Geometry check sheet. Reference: the model listing, model coordinates, mm. A direction names the side the tool comes from. Coordinates: 2 decimals unless noted, no trailing zeros. Loops run counter-clockwise (first coordinate to the right, second up) from the corner with the lowest first, then second, coordinate; pieces in that order, holes last. Notation, with made-up numbers: M 49.25,-24.5 L 105.25,-24.5 A22 cw 105.25,-17.5 Z; hole C 4,5 d9. An arc over 180 degrees is marked long. Use CSV: the item, a comma, the result in double quotes.
```python
from build123d import *

# Parameters (mm, degrees)
F0_R     = 25.4
F0_W     = 3.81
F0_H     = 19.05
F1_DEPTH = 3.429


# Not quite as in the source:
# - ends of sketch curves that miss each other by under 0.0002 mm in the source are joined


with BuildPart() as f1:
    # F0 (on Front) → F1 (new body)
    with BuildSketch(Plane.XZ):
        with BuildLine():
            ThreePointArc((-642.1692497265, -473.1768646252), (-619.4825639758, -474.3339275445), (-599.5683960075, -485.2632650852))
            ThreePointArc((-599.5683960075, -485.2632650852), (-473.9081608396, -561.5426017902), (-329.3321582, -588.1285164))
            Line((-329.3321582, -588.1285164), (312.391679, -588.1285164))
            ThreePointArc((312.391679, -588.1285164), (370.7126340924, -576.5277571547), (420.1547524528, -543.4915898528))
            Line((420.1547524528, -543.4915898528), (432.6678418, -530.9785164))
            Line((432.6678418, -530.9785164), (432.6678418, -518.2785164))
            Line((432.6678418, -518.2785164), (115.1678418, -518.2785164))
            Line((115.1678418, -518.2785164), (115.1678418, -486.5285164))
            Line((115.1678418, -486.5285164), (-329.3321582, -486.5285164))
            ThreePointArc((-329.3321582, -486.5285164), (-500.4183293998, -433.9834708096), (-612.5167665735, -294.4650126217))
            Line((-612.5167665735, -294.4650126217), (-633.7122454, -241.2238))
            ThreePointArc((-633.7122454, -241.2238), (-715.4828245955, -108.0397407431), (-837.3321571082, -10.1767620246))
            Line((-837.3321571082, -10.1767620246), (-888.1321582, -98.1649548))
            ThreePointArc((-888.1321582, -98.1649548), (-792.2711581527, -174.5413586603), (-728.0333576386, -278.9261845185))
            Line((-728.0333576386, -278.9261845185), (-706.971662, -331.8929862))
            ThreePointArc((-706.971662, -331.8929862), (-701.288086285, -345.465340488), (-695.1169115223, -358.8230511462))
            ThreePointArc((-695.1169115223, -358.8230511462), (-695.6103607346, -404.0881567784), (-732.0186808394, -430.9880994311))
            Line((-732.0186808394, -430.9880994311), (-778.7941498, -439.2359008))
            ThreePointArc((-778.7941498, -439.2359008), (-797.5979576606, -451.5111596623), (-801.724697479, -473.5845717908))
            Line((-801.724697479, -473.5845717908), (-659.172037, -448.448684))
            Line((-659.172037, -448.448684), (-658.5104432, -452.2007974))
            Line((-658.5104432, -452.2007974), (-800.6426456, -477.2625456))
            ThreePointArc((-800.6426456, -477.2625456), (-788.0677244467, -492.1533513081), (-768.8701676538, -495.5176466233))
            Line((-768.8701676538, -495.5176466233), (-642.1692497265, -473.1768646252))
        make_face()
        Polygon((-753.9383956, -462.4504086), (-757.24639, -443.6898162), (-750.74272, -442.543057), (-747.4347256, -461.3036494), align=None, mode=Mode.SUBTRACT)
        with Locations((-562.9950386, -449.5436526)):
            Circle(F0_R, mode=Mode.SUBTRACT)
        with Locations((-431.0197374, -522.7745704)):
            Circle(F0_R, mode=Mode.SUBTRACT)
        with Locations((-349.0011308, -536.6188658)):
            Circle(F0_R, mode=Mode.SUBTRACT)
        Polygon((-383.0809204, -523.6095192), (-386.1430682, -542.411793), (-389.9035128, -541.7993482), (-386.841365, -522.9970744), align=None, mode=Mode.SUBTRACT)
        with Locations((-279.3916688, -536.6188658)):
            Circle(F0_R, mode=Mode.SUBTRACT)
        with Locations((-500.8834026, -493.095026)):
            Circle(F0_R, mode=Mode.SUBTRACT)
        Polygon((-590.2629546, -409.075509), (-604.6945742, -421.510587), (-607.1815898, -418.624258), (-592.7499702, -406.1892054), align=None, mode=Mode.SUBTRACT)
        with Locations((-618.3772494, -388.5352402)):
            Circle(F0_R, mode=Mode.SUBTRACT)
        with Locations((-652.7354484, -328.9401854)):
            Circle(F0_R, mode=Mode.SUBTRACT)
        with Locations((-209.7308988, -536.6188658)):
            Circle(F0_R, mode=Mode.SUBTRACT)
        with Locations((-176.9321582, -537.3285164)):
            Rectangle(F0_W, F0_H, mode=Mode.SUBTRACT)
        with Locations((62.7803418, -537.3285164)):
            Rectangle(F0_W, F0_H, mode=Mode.SUBTRACT)
        with Locations((-678.731434, -265.7196362)):
            Circle(F0_R, mode=Mode.SUBTRACT)
        Polygon((-683.8231434, -229.7111992), (-700.9451564, -238.0621858), (-702.6153588, -234.6377832), (-685.4933458, -226.2867966), align=None, mode=Mode.SUBTRACT)
        with Locations((-713.8615898, -194.4801292)):
            Circle(F0_R, mode=Mode.SUBTRACT)
        with Locations((-760.120654, -134.1457058)):
            Circle(F0_R, mode=Mode.SUBTRACT)
        with Locations((-811.7017548, -87.0353098)):
            Circle(F0_R, mode=Mode.SUBTRACT)
    extrude(amount=F1_DEPTH)


solid = f1.part
```
1. Thickness scan on line 1 (X direction, y = -1, z = -407); line 2 (X direction, y = -0.6, z = -221); line 3 (X direction, y = -1.9, z = -143). Record the ranges inside material, lowest first. Write a range as [from, to].
The answers:
line 1,"[-697.22, -635.82], [-600.94, -593.69], [-592.05, -534.65]"
line 2,"[-757.45, -642.33]"
line 3,"[-823.96, -783.93], [-736.31, -687.59]"
2. Section check D-D, the plane x = 334. Record the cut outline in (y, z), plus the area to 3 significant figures.
The answers:
outline,"M -3.43,-586.59 L 0,-586.59 L 0,-518.28 L -3.43,-518.28 Z"
area,"234 mm^2"
3. Section check B-B, the plane y = -1.6. Count the separate pieces of the cut face and the enclosed holes in it, plus the area to 3 significant figures.
The answers:
separate pieces,"1"
enclosed holes,"18"
area,"128,000 mm^2"
4. Section check A-A, the plane x = -554. Record the cut outline in (y, z).
The answers:
outline,"M -3.43,-520.38 L 0,-520.38 L 0,-473.3 L -3.43,-473.3 Z; M -3.43,-425.79 L 0,-425.79 L 0,-387.71 L -3.43,-387.71 Z"
5. Release check for a two-part mould opening along Z. For faces 1 (the cylindrical face through (-498.31, -1.69, -435.4)), 2 (the flat face through (-329, 0, -490)), 3 (the cylindrical face through (-639.081, -1.69, -307.523)) record: +Z half, -Z half, draft (parallel to the pull), parting line (faces both ways), or undercut.
The answers:
face 1,"+Z half"
face 2,"draft"
face 3,"undercut"
6. Section check C-C, the plane x = -152.5. Record the cut outline in (y, z), plus the area to 3 significant figures.
The answers:
outline,"M -3.43,-588.13 L 0,-588.13 L 0,-486.53 L -3.43,-486.53 Z"
area,"348 mm^2"
7. Gauge pin test, flat ends, axial feed: P1, Ø1.7, axis at x = 257, y = -2, coming from the +Z side; P2, Ø1.7, axis at y = -2, z = -535.5, coming from the +X side; P3, Ø1, axis at y = -1.5, z = -535, coming from the -X side. Record the tip position at first contact, or that the pin passes through.
The answers:
P1,"z = -518.28"
P2,"x = 429"
P3,"x = -531.11"
8. Set-up check for faces 4 (the cylindrical face through (-793.42, -1.69, -173.25)), 5 (the flat face through (-731.446, -1.69, -461.193)), 6 (the flat face through (-706.407, -1.69, -484.504)): record each of +Z, -Z, +X, -X, +Y, -Y from which the full face is reachable in a straight line by a thin tool's end or side.
The answers:
face 4,"-X, +Y, -Y"
face 5,"+Y, -Y"
face 6,"-Z, +Y, -Y"
